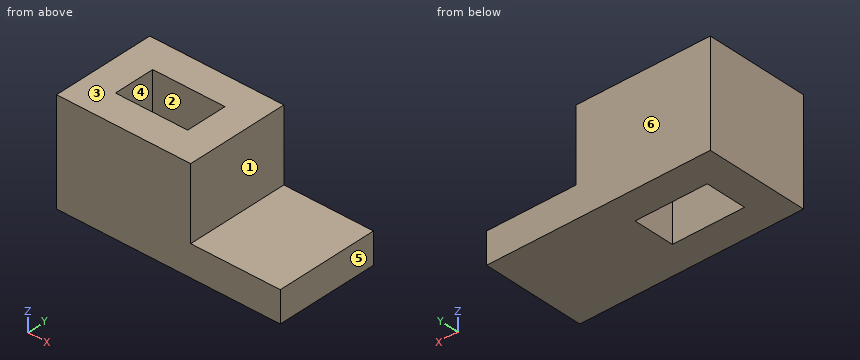
from build123d import *

# Parameters (mm, degrees)
F0_W     = 82.55
F0_H     = 63.5
F1_DEPTH = 63.5
F0_W_2   = 55.153496
F2_DEPTH = 19.05
F4_DEPTH = 63.501


with BuildPart() as f1:
    # F0 (on Top) → F1 (new body)
    with BuildSketch(Plane.XY):
        with Locations((-41.275, 31.75)):
            Rectangle(F0_W, F0_H)
    extrude(amount=F1_DEPTH)

    # F0 (on Top) → F2 (join)
    with BuildSketch(Plane.XY):
        with Locations((27.576748, 31.75)):
            Rectangle(F0_W_2, F0_H)
    extrude(amount=F2_DEPTH)

    # F3 (on face) → F4 (cut, through all)
    with BuildSketch(Plane.XY.offset(63.5)):
        Polygon((-63.5, 44.45), (-63.5, 31.75), (-63.5, 19.05), (-41.275, 19.05), (-19.05, 19.05), (-19.05, 31.75), (-19.05, 44.45), (-41.275, 44.45), align=None)
    extrude(amount=-F4_DEPTH, mode=Mode.SUBTRACT)


solid = f1.part
The model under review builds one solid part; all positions refer to its coordinate system, in mm. Face numbers are marked on the shaded views. A direction names the side the tool comes from. Give positions to 0.01 mm unless a question says otherwise; leave off trailing zeros. Write each loop counter-clockwise with the first axis right and the second up, starting at its lowest first coordinate (ties: lowest second). Pieces come first, ordered by that corner, then holes. Notation, with made-up numbers: M 73.5,42 L 127.5,42 A6 ccw 127.5,49 Z; hole C 72.25,-38.75 d11. An arc over 180 degrees is marked long. One line per question, with ' | ' between items. Start each with the question number.
Item 1: We need section B-B on x = -40. Write out the cut boundary in (y, z).
Item 2: Draft analysis for pull direction X (two halves, no side actions). For the marked faces 4, 5 and 6, state which applies: released by +X, released by -X, zero draft, split by the parting line, or undercut.
Item 3: For pin 1 (22 mm diameter, centred on y = 31.5, z = 45.5, fed in from +X), flat-tipped, find the tip position at first contact; note if it passes through.
Item 4: Wall thickness on line 1 (X direction, y = 24.5, z = 51); line 2 (X direction, y = 29, z = 13); line 3 (Y direction, x = -20.5, z = 30.5): over which ranges is each line inside the solid? List them lowest first. Write a range as from..to.
Item 5: We need section A-A on y = 36. Write out the cut boundary in (x, z), plus the area to 3 significant figures.
Item 6: For the marked faces 1, 2 and 3, list the 3-axis set-ups (+Z, -Z, +X, -X, +Y, -Y) from which the entire face can be reached by the end or side of a thin tool; tool diameter is ignored.
Item 7: We need section D-D on z = 17. Write out the cut boundary in (x, y), plus the area to 3 significant figures.
Item 8: We need section C-C on z = 26. Write out the cut boundary in (x, y).
Results found:
1) outline: M 0,0 L 19.05,0 L 19.05,63.5 L 0,63.5 Z; M 44.45,0 L 63.5,0 L 63.5,63.5 L 44.45,63.5 Z
2) face 4: undercut | face 5: released by +X | face 6: zero draft
3) pin 1: stops at x = 0
4) line 1: x = -82.55..-63.5, -19.05..0 | line 2: x = -82.55..-63.5, -19.05..55.15 | line 3: y = 0..19.05, 44.45..63.5
5) outline: M -82.55,0 L -63.5,0 L -63.5,63.5 L -82.55,63.5 Z; M -19.05,0 L 55.15,0 L 55.15,19.05 L 0,19.05 L 0,63.5 L -19.05,63.5 Z | area: 3,470 mm2
6) face 1: +Z, +X, +Y, -Y | face 2: +Z, -Z | face 3: +Z, +X, -X, +Y, -Y
7) outline: M -82.55,0 L 55.15,0 L 55.15,63.5 L -82.55,63.5 Z; hole M -63.5,19.05 L -19.05,19.05 L -19.05,44.45 L -63.5,44.45 Z | area: 7,620 mm2
8) outline: M -82.55,0 L 0,0 L 0,63.5 L -82.55,63.5 Z; hole M -63.5,19.05 L -19.05,19.05 L -19.05,44.45 L -63.5,44.45 Z
